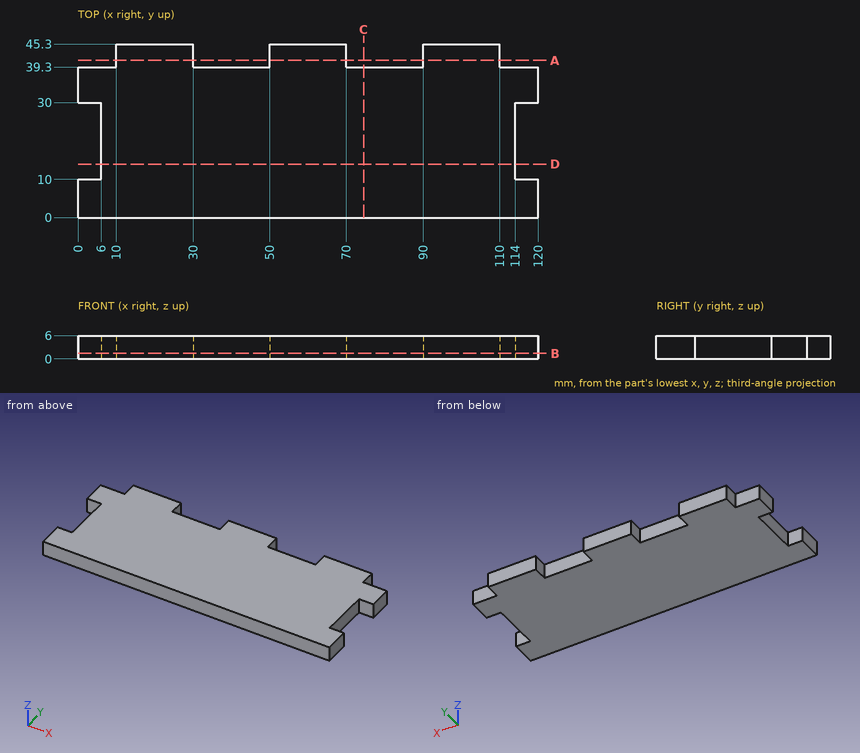
Input: dimensioned drawing with shaded views. Units: mm. Origin: part minimum x, y, z. Round coordinates to 2 decimals unless told otherwise and drop trailing zeros. Order: outer loops, then holes, each group sorted by start corner. A loop starts at its lowest first (then second) coordinate and runs counter-clockwise, first axis right, second up.
Q1. Section B-B, the plane z = 1.4. Output: boundary loops of the cut face in (x, y).
Result sheet:
outline: (0, 0) - (120, 0) - (120, 10) - (114, 10) - (114, 30) - (120, 30) - (120, 39.3) - (110, 39.3) - (110, 45.3) - (90, 45.3) - (90, 39.3) - (70, 39.3) - (70, 45.3) - (50, 45.3) - (50, 39.3) - (30, 39.3) - (30, 45.3) - (10, 45.3) - (10, 39.3) - (0, 39.3) - (0, 30) - (6, 30) - (6, 10) - (0, 10) - close
Q2. Pin query (flat end, axial travel): pin 1 (3 mm diameter, centred on x = 7.5, z = 4, fed in from +Y); pin 2 (3 mm diameter, centred on y = 42, z = 3, fed in from +X); pin 3 (3 mm diameter, centred on y = 43, z = 2.5, fed in from -X); pin 4 (10 mm diameter, centred on x = 37, y = 22, fed in from -Z). Return the tip coordinate at first contact, or that it passes through.
Result sheet:
pin 1: stops at y = 39.3
pin 2: stops at x = 110
pin 3: stops at x = 10
pin 4: stops at z = 0
Q3. Material intervals for probe 1 along X at (y, z) = (41.5, 5.35); probe 2 along X at (y, z) = (14.5, 5.2); probe 3 along Y at (x, z) = (72, 4.4), sorted ascending.
Result sheet:
probe 1: x = 10 to 30, 50 to 70, 90 to 110
probe 2: x = 6 to 114
probe 3: y = 0 to 39.3
Q4. Section C-C, the plane x = 74.5. Output: boundary loops of the cut face in (y, z), and give its area (3 significant figures).
Result sheet:
outline: (0, 0) - (39.3, 0) - (39.3, 6) - (0, 6) - close
area: 236 mm2
Q5. Section A-A, the plane y = 41. Output: boundary loops of the cut face in (x, z), and give its area (3 significant figures).
Result sheet:
outline: (10, 0) - (30, 0) - (30, 6) - (10, 6) - close; (50, 0) - (70, 0) - (70, 6) - (50, 6) - close; (90, 0) - (110, 0) - (110, 6) - (90, 6) - close
area: 360 mm2
Q6. Section D-D, the plane y = 14. Output: boundary loops of the cut face in (x, z), and give its area (3 significant figures).
Result sheet:
outline: (6, 0) - (114, 0) - (114, 6) - (6, 6) - close
area: 648 mm2
